```python
from build123d import *

# Parameters (mm, degrees)
SKETCH_1_W          = 2
SKETCH_1_H          = 4
EXTRUDE_1_DEPTH     = 2.5
SKETCH_1_3_W        = 1.5
SKETCH_1_3_H        = 1
EXTRUDE_2_DEPTH     = 1
SKETCH_1_4_W        = 2
SKETCH_1_4_H        = 4
CUT_EXTRUDE_1_DEPTH = 0.7
CHAMFER_1_SIZE      = 0.7
CHAMFER_1_SIZE_2    = 0.490145277


with BuildPart() as part:
    # 草图1 → 凸台-拉伸1 (new body)
    # profile 1 of 2: a face of its own
    with BuildSketch(Plane.XY):
        with BuildLine():
            ThreePointArc((0.75, 3), (1.457106781, 2.707106781), (1.75, 2))
            Line((1.75, 2), (1.75, -2))
            ThreePointArc((1.75, -2), (1.457106781, -2.707106781), (0.75, -3))
            Line((0.75, -3), (-0.75, -3))
            ThreePointArc((-0.75, -3), (-1.457106781, -2.707106781), (-1.75, -2))
            Line((-1.75, -2), (-1.75, 2))
            ThreePointArc((-1.75, 2), (-1.457106781, 2.707106781), (-0.75, 3))
            Line((-0.75, 3), (0.75, 3))
        make_face()
        Rectangle(SKETCH_1_W, SKETCH_1_H, mode=Mode.SUBTRACT)
    # profile 2 of 2: a face of its own
    with BuildSketch(Plane.XY):
        Rectangle(SKETCH_1_W, SKETCH_1_H)
    extrude(amount=EXTRUDE_1_DEPTH)

    # 草图1<3> → 凸台-拉伸2 (add)
    with BuildSketch(Plane.XY):
        with Locations((0, 3.5)):
            Rectangle(SKETCH_1_3_W, SKETCH_1_3_H)
        with Locations((0, -3.5)):
            Rectangle(SKETCH_1_3_W, SKETCH_1_3_H)
    extrude(amount=EXTRUDE_2_DEPTH)

    # 草图1<4> → 切除-拉伸1 (cut)
    with BuildSketch(Plane.XY):
        Rectangle(SKETCH_1_4_W, SKETCH_1_4_H)
    extrude(amount=CUT_EXTRUDE_1_DEPTH, mode=Mode.SUBTRACT)

    # 倒角1
    # the kernel refuses this chamfer: 0.7, 0.490145277 mm, written as the material it adds along each edge
    with BuildSketch(Plane(origin=(1, -2, 0.7), x_dir=(0, -0.02220967419845705, -0.99975333476413), z_dir=(-1, 0, 0)), Plane(origin=(-1, 2, 0.7), x_dir=(0, 0.02220967419845705, -0.99975333476413), z_dir=(1, 0, 0))) as chamfer_1_piece_1:
        Polygon((CHAMFER_1_SIZE * 0.999753334764, -CHAMFER_1_SIZE * 0.0222096741985), (-CHAMFER_1_SIZE_2 * 0.022209674187, -CHAMFER_1_SIZE_2 * 0.999753334248), (0, 0), align=None)
    extrude(amount=2)
    with BuildSketch(Plane(origin=(-1, -2, 0.7), x_dir=(-0.02220967419845705, 0, -0.99975333476413), z_dir=(0, 1, 0)), Plane(origin=(1, 2, 0.7), x_dir=(0.02220967419845705, 0, -0.99975333476413), z_dir=(0, -1, 0))) as chamfer_1_piece_2:
        Polygon((CHAMFER_1_SIZE * 0.999753334764, -CHAMFER_1_SIZE * 0.0222096741985), (-CHAMFER_1_SIZE_2 * 0.022209674187, -CHAMFER_1_SIZE_2 * 0.999753334248), (0, 0), align=None)
    extrude(amount=4)


solid = part.part
```
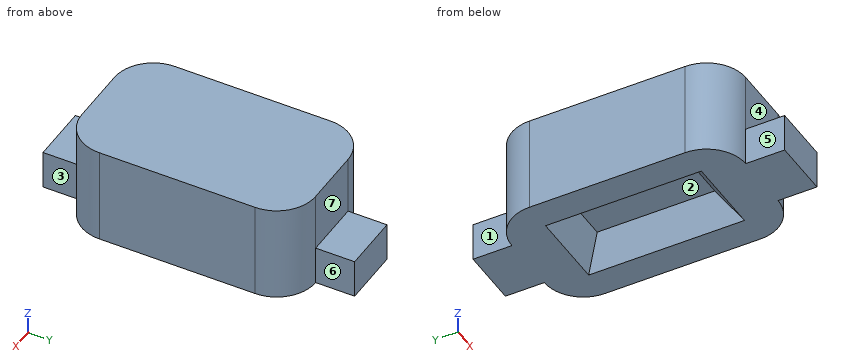
Input: part model. Units: mm. Frame: model coordinates. Face numbers are marked on the shaded views. A direction names the side the tool comes from. Coordinates: 2 decimals unless noted, no trailing zeros. Write each loop counter-clockwise with the first axis right and the second up, starting at its lowest first coordinate (ties: lowest second). Pieces come first, ordered by that corner, then holes.
1) Pin query (flat end, axial travel): pin 1 Ø0.5 at (x, y) = (0, 3.5) entering from +Z; pin 2 Ø0.5 at (y, z) = (3.5, 0.5) entering from +X; pin 3 Ø1.2 at (x, z) = (0, 2) entering from -Y. Return the tip coordinate at first contact, or that it passes through.
2) Section D-D on z = 0.85. Output: boundary loops of the cut face in (x, y).
3) Set-up query: the marked faces 4, 5, 6 and 7. Return all of +Z, -Z, +X, -X, +Y, -Y with unobstructed straight access to the full face (end or side cutting, diameter ignored); none if empty.
4) Mould query, pull axis X, two halves, no side actions, for the marked faces 1, 2 and 3. Classes: pulls with the +X half, pulls with the -X half, needs draft (parallel to the pull), parting line crosses it, or undercut.
5) Section A-A on z = 1.8. Output: boundary loops of the cut face in (x, y).
6) Material intervals for line 1 along Z through (x, y) = (-0.3, -3.5); line 2 along Z through (x, y) = (-0.3, 0.25); line 3 along Y through (x, z) = (-0.2, 2.05), sorted ascending.
7) Section C-C on y = -1. Output: boundary loops of the cut face in (x, z), and give its area (3 significant figures).
8) Section B-B on x = 0. Output: boundary loops of the cut face in (y, z).
Check result:
1. pin 1: stops at z = 1
1. pin 2: stops at x = 0.75
1. pin 3: stops at y = -3
2. outline: (-1.75, -2) arc R1 ccw to (-0.75, -3) - (-0.75, -4) - (0.75, -4) - (0.75, -3) arc R1 ccw to (1.75, -2) - (1.75, 2) arc R1 ccw to (0.75, 3) - (0.75, 4) - (-0.75, 4) - (-0.75, 3) arc R1 ccw to (-1.75, 2) - close
3. face 4: +Z, +X, -X, -Y
3. face 5: +Z, -Z, -X, -Y
3. face 6: +Z, -Z, +X, +Y
3. face 7: +Z, +X, -X, +Y
4. face 1: pulls with the -X half
4. face 2: undercut
4. face 3: pulls with the +X half
5. outline: (-1.75, -2) arc R1 ccw to (-0.75, -3) - (0.75, -3) arc R1 ccw to (1.75, -2) - (1.75, 2) arc R1 ccw to (0.75, 3) - (-0.75, 3) arc R1 ccw to (-1.75, 2) - close
6. line 1: z = 0 to 1
6. line 2: z = 0.7 to 2.5
6. line 3: y = -3 to 3
7. outline: (-1.75, 0) - (-1, 0) - (-0.51, 0.7) - (0.51, 0.7) - (1, 0) - (1.75, 0) - (1.75, 2.5) - (-1.75, 2.5) - close
7. area: 7.69 mm2
8. outline: (-4, 0) - (-2, 0) - (-1.51, 0.7) - (1.51, 0.7) - (2, 0) - (4, 0) - (4, 1) - (3, 1) - (3, 2.5) - (-3, 2.5) - (-3, 1) - (-4, 1) - close
